from build123d import *

# Parameters (mm, degrees)
F1_DEPTH = 80


with BuildPart() as f1:
    # F0 (on Top) → F1 (new body)
    with BuildSketch(Plane.XY):
        Polygon((0, 7), (0, 0), (7, 0), (7, 5.5), (13, 5.5), (13, 0), (20, 0), (20, 7), (14.5, 7), (14.5, 13), (20, 13), (20, 20), (13, 20), (13, 14.5), (7, 14.5), (7, 20), (0, 20), (0, 13), (5.5, 13), (5.5, 7), align=None)
        Polygon((7, 0), (0, 0), (0, -7), (5.5, -7), (5.5, -13), (0, -13), (0, -20), (7, -20), (7, -14.5), (13, -14.5), (13, -20), (20, -20), (20, -13), (14.5, -13), (14.5, -7), (20, -7), (20, 0), (13, 0), (13, -5.5), (7, -5.5), align=None)
    extrude(amount=F1_DEPTH)


solid = f1.part
Source: CAD feature listing. Evaluate the final solid. Frame: model axes, mm. A direction names the side the tool comes from. Give positions to 0.01 mm unless a question says otherwise; leave off trailing zeros. Write each loop counter-clockwise with the first axis right and the second up, starting at its lowest first coordinate (ties: lowest second). Pieces come first, ordered by that corner, then holes. Notation, with made-up numbers: M 27,-2.5 L 79,-2.5 A12 cw 79,7.5 Z; hole C 52.25,-16.75 d10. An arc over 180 degrees is marked long. Return JSON: item names as keys, results as strings. Group by question number.
1) Cut plane B-B, the plane y = 2. Output: boundary loops of the cut face in (x, z).
2) First-contact query: pin 1 Ø1.8 at (y, z) = (-9.5, 57.5) entering from -X; pin 2 Ø1.8 at (x, z) = (11, 55) entering from -Y; pin 3 Ø1.8 at (y, z) = (-10.5, 56.5) entering from +X. Flat tips, straight axial feed; report the tip coordinate or a pass-through.
3) Ray query, L1, parallel to Y at x = 5, z = 15.5; L2, parallel to Y at x = 10, z = 62; L3, parallel to X at y = 0, z = 56.5. Return the intervals inside material, ascending.
4) Draft query along Y for faces 4 (the face through (20, -17, 39)), 5 (the face through (10, -14.5, 39)), 6 (the face through (10, 5.5, 39)). Return one class per face: released by +Y, released by -Y, zero draft, split by the parting line, or undercut.
5) Cut plane C-C, the plane x = 17. Output: boundary loops of the cut face in (y, z), then the cut area to 3 significant figures.
6) Cut plane A-A, the plane x = 9.5. Output: boundary loops of the cut face in (y, z), then the cut area to 3 significant figures.
7) Set-up query: faces 1 (the face through (10, 14.5, 39)), 2 (the face through (7, 0, 39)), 3 (the face through (14.5, -10, 39)). Return all of +Z, -Z, +X, -X, +Y, -Y with unobstructed straight access to the full face (end or side cutting, diameter ignored); none if empty.
Data:
{
 "1": {"outline": "M 0,0 L 7,0 L 7,80 L 0,80 Z; M 13,0 L 20,0 L 20,80 L 13,80 Z"},
 "2": {"pin 1": "stops at x = 5.5", "pin 2": "stops at y = -14.5", "pin 3": "stops at x = 14.5"},
 "3": {"L1": "y = -20 to -13, -7 to 7, 13 to 20", "L2": "y = -14.5 to -5.5, 5.5 to 14.5", "L3": "x = 0 to 7, 13 to 20"},
 "4": {"face 4": "zero draft", "face 5": "released by -Y", "face 6": "undercut"},
 "5": {"outline": "M -20,0 L -13,0 L -13,80 L -20,80 Z; M -7,0 L 7,0 L 7,80 L -7,80 Z; M 13,0 L 20,0 L 20,80 L 13,80 Z", "area": "2,240 mm²"},
 "6": {"outline": "M -14.5,0 L -5.5,0 L -5.5,80 L -14.5,80 Z; M 5.5,0 L 14.5,0 L 14.5,80 L 5.5,80 Z", "area": "1,440 mm²"},
 "7": {"face 1": "+Z, -Z, +Y", "face 2": "+Z, -Z", "face 3": "+Z, -Z, +X"}
}
